For this review, take the finished solid that the model builds, in its own axes (mm). Face numbers are marked on the shaded views. Coordinates: 2 decimals unless noted, no trailing zeros. Loops run counter-clockwise (first coordinate to the right, second up) from the corner with the lowest first, then second, coordinate; pieces in that order, holes last.
1. To check wall thickness, follow probe 1 along Z at (x, y) = (-25, -4.25); probe 2 along Z at (x, y) = (-27, 7.75); probe 3 along Z at (x, y) = (5, -1.75). State the ranges of each line that lie inside material, in increasing order.
2. Take a section at B-B, the plane z = 0. State the section outline as (x, y) points (3 decimals), then the cut area to 3 significant figures.
3. Mouldability with a two-part tool opening along Z and no side actions: class the marked faces 1, 2, 3 and 4 as pulls with the +Z half, pulls with the -Z half, needs draft (parallel to the pull), parting line crosses it, or undercut.
4. Clearance check with flat-ended pins moving along their axes: P1, Ø6.5, axis at x = -25.98, z = 15, coming from the +Y side; P2, Ø20, axis at x = 0.5, z = 0.5, coming from the -Y side; P3, Ø10, axis at x = -28, y = 1, coming from the +Z side; P4, Ø2, axis at y = 7.5, z = 0.5, coming from the -X side. State where each tip first meets the part, or that it passes through.
5. Take a section at D-D, the plane z = 15. State the section outline as (x, y) points.
6. Take a section at C-C, the plane y = -2. State the section outline as (x, z) points.
7. Take a section at A-A, the plane x = 0. State the section outline as (y, z) points (3 decimals), then the cut area to 3 significant figures.
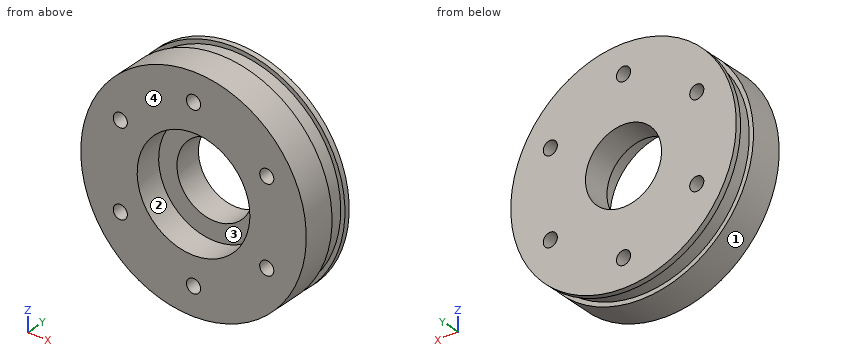
```python
from build123d import *

# Parameters (mm, degrees)
SKETCH1_R                = 38.515
BOSS_EXTRUDE1_DEPTH      = 10
SKETCH2_R                = 40
BOSS_EXTRUDE2_DEPTH      = 2
BOSS_EXTRUDE3_DEPTH      = 10
BOSS_EXTRUDE3_DEPTH_BACK = 2
SKETCH3_R                = 40
SKETCH4_R                = 13.5
SKETCH4_R_2              = 2.5
CUT_EXTRUDE1_DEPTH       = 61
SKETCH5_R                = 20
CUT_EXTRUDE2_DEPTH       = 10


with BuildPart() as part:
    # Sketch1 → Boss-Extrude1 (new body)
    with BuildSketch(Plane(origin=(0, 0, 0), x_dir=(1, 0, 0), z_dir=(0, 1, 0))):
        with Locations(Location((0, 0, 0), (0, 0, 270))):
            Circle(SKETCH1_R)
    extrude(amount=BOSS_EXTRUDE1_DEPTH)

    # Sketch2 → Boss-Extrude2 (add)
    with BuildSketch(Plane(origin=(0, 10, 0), x_dir=(1, 0, 0), z_dir=(0, 1, 0))):
        with Locations(Location((0, 0, 0), (0, 0, 270))):
            Circle(SKETCH2_R)
    extrude(amount=-BOSS_EXTRUDE2_DEPTH)

    # Sketch3 → Boss-Extrude3 (add, two sides: drawn at the far end of the back side and taken through both)
    with BuildSketch(Plane.XZ.offset(-BOSS_EXTRUDE3_DEPTH_BACK)):
        with Locations(Location((0, 0, 0), (0, 0, 90))):
            Circle(SKETCH3_R)
    extrude(amount=BOSS_EXTRUDE3_DEPTH + BOSS_EXTRUDE3_DEPTH_BACK)

    # Sketch4 → Cut-Extrude1 (cut, through all)
    with BuildSketch(Plane.XZ.offset(10)):
        with Locations(Location((0, 0, 0), (0, 0, 270))):
            Circle(SKETCH4_R)
        with Locations(Location((0, 30, 0), (0, 0, 270))):
            Circle(SKETCH4_R_2)
        with Locations(Location((25.980762114, 15, 0), (0, 0, 270))):
            Circle(SKETCH4_R_2)
        with Locations(Location((25.980762114, -15, 0), (0, 0, 270))):
            Circle(SKETCH4_R_2)
        with Locations(Location((0, -30, 0), (0, 0, 270))):
            Circle(SKETCH4_R_2)
        with Locations(Location((-25.980762114, -15, 0), (0, 0, 270))):
            Circle(SKETCH4_R_2)
        with Locations(Location((-25.980762114, 15, 0), (0, 0, 270))):
            Circle(SKETCH4_R_2)
    extrude(amount=-CUT_EXTRUDE1_DEPTH, mode=Mode.SUBTRACT)

    # Sketch5 → Cut-Extrude2 (cut)
    with BuildSketch(Plane.XZ.offset(10)):
        with Locations(Location((0, 0, 0), (0, 0, 270))):
            Circle(SKETCH5_R)
    extrude(amount=-CUT_EXTRUDE2_DEPTH, mode=Mode.SUBTRACT)


solid = part.part
```
Results list:
1. probe 1: z = -31.22 to -17.3, -12.7 to 12.7, 17.3 to 31.22
1. probe 2: z = -27.47 to -17.28, -12.72 to 12.72, 17.28 to 27.47
1. probe 3: z = -39.69 to -19.36, 19.36 to 39.69
2. outline: (-40, -10) - (-20, -10) - (-20, 0) - (-13.5, 0) - (-13.5, 10) - (-40, 10) - (-40, 8) - (-38.515, 8) - (-38.515, 2) - (-40, 2) - close; (13.5, 0) - (20, 0) - (20, -10) - (40, -10) - (40, 2) - (38.515, 2) - (38.515, 8) - (40, 8) - (40, 10) - (13.5, 10) - close
2. area: 912 mm2
3. face 1: parting line crosses it
3. face 2: undercut
3. face 3: undercut
3. face 4: needs draft
4. P1: stops at y = 10
4. P2: passes through
4. P3: stops at z = 32.73
4. P4: stops at x = -40
5. outline: (-37.08, -10) - (-28.48, -10) - (-28.48, 10) - (-37.08, 10) - (-37.08, 8) - (-35.47, 8) - (-35.47, 2) - (-37.08, 2) - close; (-23.48, -10) - (-13.23, -10) - (-13.23, 0) - (13.23, 0) - (13.23, -10) - (23.48, -10) - (23.48, 10) - (-23.48, 10) - close; (28.48, -10) - (37.08, -10) - (37.08, 2) - (35.47, 2) - (35.47, 8) - (37.08, 8) - (37.08, 10) - (28.48, 10) - close
6. outline: circle Ø80 at (0, 0); hole circle Ø5 at (-25.98, -15); hole circle Ø5 at (-25.98, 15); hole circle Ø40 at (0, 0); hole circle Ø5 at (0, -30); hole circle Ø5 at (0, 30); hole circle Ø5 at (25.98, -15); hole circle Ø5 at (25.98, 15)
7. outline: (-10, -40) - (2, -40) - (2, -38.515) - (8, -38.515) - (8, -40) - (10, -40) - (10, -32.5) - (-10, -32.5) - close; (-10, -27.5) - (10, -27.5) - (10, -13.5) - (0, -13.5) - (0, -20) - (-10, -20) - close; (-10, 20) - (0, 20) - (0, 13.5) - (10, 13.5) - (10, 27.5) - (-10, 27.5) - close; (-10, 32.5) - (10, 32.5) - (10, 40) - (8, 40) - (8, 38.515) - (2, 38.515) - (2, 40) - (-10, 40) - close
7. area: 712 mm2
